```python
from build123d import *

# Parameters (mm, degrees)
SKETCH1_R           = 2.5
BOSS_EXTRUDE1_DEPTH = 5
SKETCH2_W           = 8.660254038
SKETCH2_H           = 5
BOSS_EXTRUDE2_DEPTH = 11
SKETCH3_R           = 7.5
BOSS_EXTRUDE3_DEPTH = 5
SKETCH4_R           = 2.65
CUT_EXTRUDE1_DEPTH  = 36.309767636


with BuildPart() as part:
    # Sketch1 → Boss-Extrude1 (new body)
    with BuildSketch(Plane.XY.offset(2.596184677)):
        with Locations((21.004809472, 129.315154096)):
            Circle(SKETCH1_R)
    extrude(amount=-BOSS_EXTRUDE1_DEPTH)

    # Sketch2 → Boss-Extrude2 (add)
    with BuildSketch(Plane.XY.offset(2.596184677)):
        with Locations((21.004809472, 129.315154096)):
            Rectangle(SKETCH2_W, SKETCH2_H)
    extrude(amount=BOSS_EXTRUDE2_DEPTH)

    # Sketch3 → Boss-Extrude3 (add)
    with BuildSketch(Plane(origin=(0, 131.815154096, 0), x_dir=(1, 0, 0), z_dir=(0, 1, 0))):
        with Locations((21.004809472, -12.730064941)):
            Circle(SKETCH3_R)
    extrude(amount=-BOSS_EXTRUDE3_DEPTH)

    # Sketch4 → Cut-Extrude1 (cut, through all)
    with BuildSketch(Plane(origin=(0, 131.815154096, 0), x_dir=(1, 0, 0), z_dir=(0, 1, 0))):
        with Locations(Location((21.004809472, -12.730064941, 0), (0, 0, 270))):
            Circle(SKETCH4_R)
    extrude(amount=-CUT_EXTRUDE1_DEPTH, mode=Mode.SUBTRACT)


with BuildPart() as part_1:
    # Body-Move/Copy1: moved
    add(part.part.moved(Location((-21, -129.32, -12.73))))


solid = part_1.part
```
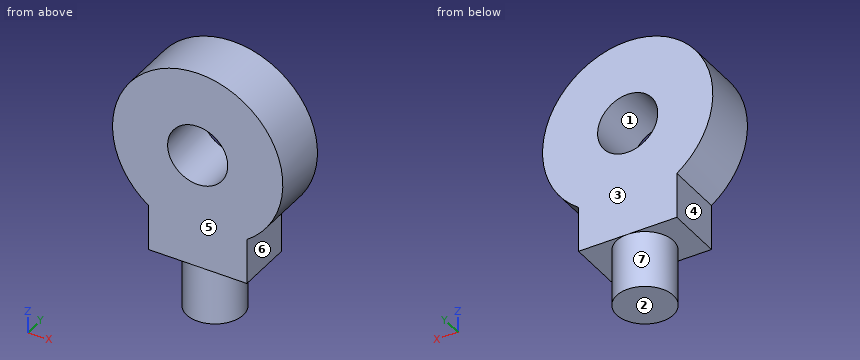
Here's how the part is built. I have some questions about the finished solid (model axes, mm). Face numbers are marked on the shaded views. A direction names the side the tool comes from. Round coordinates to 2 decimals unless told otherwise and drop trailing zeros. Order: outer loops, then holes, each group sorted by start corner. A loop starts at its lowest first (then second) coordinate and runs counter-clockwise, first axis right, second up. Notation, with made-up numbers: (86, -24) -> (93, -24) arc R14 cw to (93, -3) -> close; hole circle Ø10 at (67.5, 71.5). An arc over 180 degrees is marked (long way). Use a Markdown table: item, result. Add a question column.
(1) Suppose I cut it at D-D, the plane z = 1.25. Please give me the cut outline in (x, y).
(2) For the marked faces 4, 5, 6 and 7, which set-ups out of +Z, -Z, +X, -X, +Y, -Y let a thin tool reach every point of the face, with its end or its side?
(3) For pin 1 Ø1.5 at (x, y) = (1.5, 0.5) entering from +Z; pin 2 Ø1.2 at (y, z) = (0.5, -9) entering from -X, each with a flat end and sliding along its axis, tell me the tip position at first contact or that it passes through.
(4) Suppose I cut it at C-C, the plane y = 1.3. Please give me the cut outline in (x, z), and give its area (3 significant figures).
(5) I need wall thicknesses on line 1 along Z through (x, y) = (0, -0.25); line 2 along X through (y, z) = (0.1, -7); line 3 along X through (y, z) = (2.1, 1). Which ranges of each line are inside material? Lowest first, please.
(6) Suppose I cut it at B-B, the plane z = -1.5. Please give me the cut outline in (x, y).
(7) If we mould it in two halves opening along Z, with no side actions, what happens to the marked faces 1, 2 and 3? For each: released by +Z, released by -Z, zero draft, split by the parting line, or undercut.
Verdict:
| question | item | result |
|---|---|---|
| 1 | outline | (-7.39, -2.5) -> (-2.33, -2.5) -> (-2.33, 2.5) -> (-7.39, 2.5) -> close; (2.34, -2.5) -> (7.4, -2.5) -> (7.4, 2.5) -> (2.34, 2.5) -> close |
| 2 | face 4 | -Z, -X, +Y, -Y |
| 2 | face 5 | +Z, -Z, +X, -X, -Y |
| 2 | face 6 | -Z, +X, +Y, -Y |
| 2 | face 7 | -Z |
| 3 | pin 1 | z = 7.46 |
| 3 | pin 2 | x = -4.33 |
| 4 | outline | (-4.33, -10.13) -> (-2.13, -10.13) -> (-2.13, -15.13) -> (2.14, -15.13) -> (2.14, -10.13) -> (4.33, -10.13) -> (4.33, -6.12) arc R7.5 ccw (long way) to (-4.33, -6.12) -> close; hole circle Ø5.3 at (0, 0) |
| 4 | area | 203 mm2 |
| 5 | line 1 | -15.13 to -2.65, 2.65 to 7.5 |
| 5 | line 2 | -4.33 to 4.33 |
| 5 | line 3 | -7.43 to -2.45, 2.46 to 7.44 |
| 6 | outline | (-7.34, -2.5) -> (-2.18, -2.5) -> (-2.18, 2.5) -> (-7.34, 2.5) -> close; (2.19, -2.5) -> (7.35, -2.5) -> (7.35, 2.5) -> (2.19, 2.5) -> close |
| 7 | face 1 | undercut |
| 7 | face 2 | released by -Z |
| 7 | face 3 | zero draft |
